```python
from build123d import *

# Parameters (mm, degrees)
PAD_DEPTH = 1.328


with BuildPart() as part:
    # Sketch → Pad (new body, symmetric)
    with BuildSketch(Plane(origin=(78.011172, 0, 0), x_dir=(1, 0, 0), z_dir=(0, 0, -1))):
        with BuildLine():
            Line((-78.011172, 0), (214, 0))
            Line((214, 0), (214, -2))
            ThreePointArc((212, -5.464102), (213.464102, -4), (214, -2))
            Line((212, -5.464102), (173.21539, -27.856406))
            ThreePointArc((165.21539, -30), (169.356495, -29.454813), (173.21539, -27.856406))
            Line((165.21539, -30), (-29.226562, -30))
            ThreePointArc((-37.226562, -27.856406), (-33.367667, -29.454813), (-29.226562, -30))
            Line((-37.226562, -27.856406), (-76.011172, -5.464102))
            ThreePointArc((-78.011172, -2), (-77.475274, -4), (-76.011172, -5.464102))
            Line((-78.011172, -2), (-78.011172, 0))
        make_face()
    extrude(amount=PAD_DEPTH, both=True)


solid = part.part
```
Design review of the part built by this model. Coordinates are the model's own, in mm. Give positions to 0.01 mm unless a question says otherwise; leave off trailing zeros. Write each loop counter-clockwise with the first axis right and the second up, starting at its lowest first coordinate (ties: lowest second). Pieces come first, ordered by that corner, then holes.
(1) Add section B-B (y = 18). Give the boundary of the cut face in (x, z), and give its area (3 significant figures).
Checked values:
outline: (23.71, -1.33) - (268.3, -1.33) - (268.3, 1.33) - (23.71, 1.33) - close
area: 650 mm2
(2) Clearance check with a flat-ended pin moving along its axis: pin 1 Ø1.5 at (y, z) = (25, 1) entering from -X. State where the tip first meets the part, or that it passes through.
Checked values:
pin 1: stops at x = 34.54
(3) Add section A-A (z = -0.25). Give the boundary of the cut face in (x, y).
Checked values:
outline: (0, 0) - (292.01, 0) - (292.01, 2) arc R4 ccw to (290.01, 5.46) - (251.23, 27.86) arc R16 ccw to (243.23, 30) - (48.78, 30) arc R16 ccw to (40.78, 27.86) - (2, 5.46) arc R4 ccw to (0, 2) - close
(4) Wall thickness on line 1 along X through (y, z) = (18.5, 0.5); line 2 along Y through (x, z) = (277, 0.65); line 3 along X through (y, z) = (4, 0.4): over which ranges is each line inside the solid? List them lowest first.
Checked values:
line 1: x = 24.58 to 267.43
line 2: y = 0 to 12.98
line 3: x = 0.54 to 291.48
